from build123d import *

# Parameters (mm, degrees)
SKETCH1_W           = 304.8
SKETCH1_H           = 304.8
BOSS_EXTRUDE1_DEPTH = 3.175
SKETCH2_W           = 298.45
SKETCH2_H           = 3.175
BOSS_EXTRUDE2_DEPTH = 63.5


with BuildPart() as part:
    # Sketch1 → Boss-Extrude1 (new body)
    with BuildSketch(Plane.XY):
        with Locations((152.4, 152.4)):
            Rectangle(SKETCH1_W, SKETCH1_H)
    extrude(amount=BOSS_EXTRUDE1_DEPTH)

    # Sketch2 → Boss-Extrude2 (add)
    with BuildSketch(Plane.XY.offset(3.175)):
        with Locations((152.4, 1.5875)):
            Rectangle(SKETCH2_W, SKETCH2_H)
        Polygon((3.175, 301.625), (0, 301.625), (0, 0), (3.175, 0), (3.175, 3.175), align=None)
        Polygon((304.8, 301.625), (304.8, 304.8), (0, 304.8), (0, 301.625), (3.175, 301.625), (301.625, 301.625), align=None)
        Polygon((304.8, 0), (304.8, 301.625), (301.625, 301.625), (301.625, 3.175), (301.625, 0), align=None)
    extrude(amount=BOSS_EXTRUDE2_DEPTH)


solid = part.part
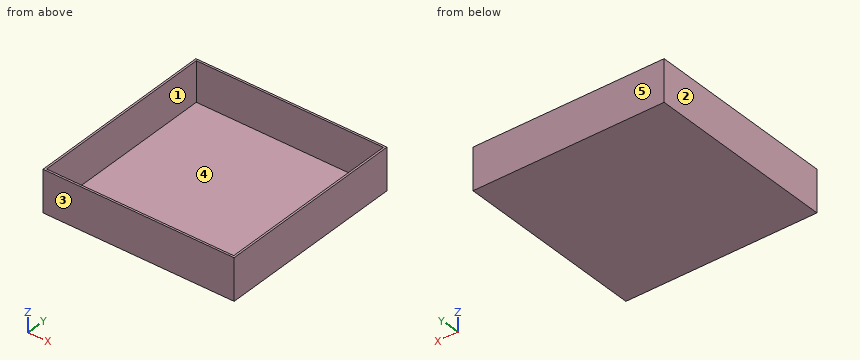
Could you check a few things on this model? Use its own coordinates, in mm. Face numbers are marked on the shaded views. A direction names the side the tool comes from. Round coordinates to 2 decimals unless told otherwise and drop trailing zeros. Order: outer loops, then holes, each group sorted by start corner. A loop starts at its lowest first (then second) coordinate and runs counter-clockwise, first axis right, second up. Notation, with made-up numbers: M -27,83.25 L 17,83.25 A30 ccw 17,107.25 Z; hole C 19,46.5 d8. An arc over 180 degrees is marked long. One line per item, written item: value.
(1) Which directions (+Z, -Z, +X, -X, +Y, -Y) give clear straight access to the entire face, cutting with the end or side of a thin tool? Please do the marked faces 4 and 5.
Ans:
face 4: +Z
face 5: +Z, -Z, +X, -X, +Y
(2) I'm going to push a flat-ended pin straight in: P1, Ø6, axis at x = 197, y = 121.5, coming from the +Z side (3 decimals). Where does the tip first touch, or does it pass through?
Ans:
P1: stops at z = 3.175
(3) Imagine slicing it at B-B (x = 168). Write out the boundary of the cut face in (y, z) (3 decimals), and give its area (3 significant figures).
Ans:
outline: M 0,0 L 304.8,0 L 304.8,66.675 L 301.625,66.675 L 301.625,3.175 L 3.175,3.175 L 3.175,66.675 L 0,66.675 Z
area: 1,370 mm^2
(4) I need wall thicknesses on line 1 along Y through (x, z) = (103.5, 47) (3 decimals); line 2 along Z through (x, y) = (254, 194) (3 decimals). Which ranges of each line are inside material? Lowest first, please. Write a range as from..to.
Ans:
line 1: y = 0..3.175, 301.625..304.8
line 2: z = 0..3.175
(5) Imagine slicing it at A-A (z = 40.5). Write out the boundary of the cut face in (x, y) (3 decimals), and give its area (3 significant figures).
Ans:
outline: M 0,0 L 304.8,0 L 304.8,304.8 L 0,304.8 Z; hole M 3.175,3.175 L 301.625,3.175 L 301.625,301.625 L 3.175,301.625 Z
area: 3,830 mm^2
(6) If we mould it in two halves opening along X, with no side actions, what happens to the marked faces 1, 2 and 3? For each: released by +X, released by -X, zero draft, split by the parting line, or undercut.
Ans:
face 1: undercut
face 2: released by -X
face 3: zero draft
